The model under review builds one solid part; all positions refer to its coordinate system, in mm. A direction names the side the tool comes from. Give positions to 0.01 mm unless a question says otherwise; leave off trailing zeros. Order: outer loops, then holes, each group sorted by start corner. A loop starts at its lowest first (then second) coordinate and runs counter-clockwise, first axis right, second up. Notation, with made-up numbers: (62.5, 62) - (121.5, 62) arc R18 ccw to (121.5, 66) - close; hole circle Ø7 at (12, -39). An arc over 180 degrees is marked (long way). Put each result on its own line as item: value.
Autodesk Inventor part; units mm, degrees
ref_plane "Work Plane1" through (11.4315, 0, 0) normal (0, 0, -1) x (-1, 0, 0)
ref_plane "YZ Plane" through (0, 0, 0) normal (1, 0, 0) x (0, 1, 0)
ref_plane "XZ Plane" through (0, 0, 0) normal (0, 1, 0) x (-1, 0, 0)
sketch "Skizze1" plane through (0, 0, 0) normal (0, 0, 1) x (1, 0, 0)
  line L0 (-0.8145, 0) -> (4.5691, 0)
  line L1 (1.1089, 2.4) -> (0.7864, 3.6035)
  line L2 (1.1089, 2.4) -> (3.8, 2.4) construction
  line L3 (3.8, 2.4) -> (3.8, 0) construction
  arc A0 (0.7864, 3.6035) -> (0, 3.5) centre (0.4, 3.5) ccw
  line L4 (1.1089, 2.4) -> (1.1089, 0)
  line L5 (0, -0.7897) -> (0, 4.738)
  point P0 (0, 0)
  dimension "d2" = 4.8
  dimension "d4" = 7.8
  dimension "d5" = 0.4
  dimension "d15" = 3.8
  dimension "d16" = 15
revolve "Ring" add sketch "Skizze1" angle 360 about axis through (-10, 0, 0) along (1, 0, 0)
sketch "Skizze2" plane through (0, 0, 0) normal (-1, 0, 0) x (0, 0, 1)
  circle A0 centre (0, 0) radius 4.9
  line L0 (-3, -1.7321) -> (-3, 1.7321)
  line L1 (-3, 1.7321) -> (0, 3.4641)
  line L2 (0, 3.4641) -> (3, 1.7321)
  line L3 (3, 1.7321) -> (3, -1.7321)
  line L4 (3, -1.7321) -> (0, -3.4641)
  line L5 (0, -3.4641) -> (-3, -1.7321)
  dimension "d55" = 6
extrude "Körper" add sketch "Skizze2" against normal blind 3 contours L0 L1 L2 L3 L4 L5
sketch "Skizze3" plane through (0, 0, 0) normal (0, 0, 1) x (1, 0, 0)
  line L0 (0.8237, 3.4641) -> (3, 3.4641)
  line L1 (3, 1.7321) -> (3, 3.4641)
  line L2 (0, -3.5) -> (0, 3.5)
  line L3 (-0.6, 0) -> (3.6, 0)
  line L4 (2.7149, 3.4641) -> (3, 2.4)
  dimension "d10" = 15
  dimension "d11" = 4.8
revolve "Fase1" cut sketch "Skizze3" angle 360 about axis through (-10, 0, 0) along (1, 0, 0)
sketch "Skizze4" plane through (0, 0, 0) normal (-1, 0, 0) x (0, 0, 1)
  circle A0 centre (0, 0) radius 3.5
hole "Gewinde" at (0, 0, 0) direction (1, 0, 0) diameter 2.459 end through all
chamfer "Fase2" distance 0.433 angle 30 1 edges at (0, 0, -1.2295) measured on face at (0, 2.7063, -0.3286)
ref_plane "Work Plane1" through (11.4315, 0, 0) normal (0, 0, -1) x (-1, 0, 0)
chamfer "Fase3" distance 0.433 angle 45 1 edges at (3, 0, -1.2295)
equation "\"d2\" = 0.6 * SW"
equation "\"d16\" = 0.6 * KEWI"
equation "\"d7\" = 0.6 * KOH"
equation "\"d10\" = ANG1"
equation "\"d11\" = 0.6 * SW0"
equation "\"d12\" = -0.5 * GD1 + 0.5 * NND"
equation "\"d46\" = -0.5 * GD1 + 0.5 * NND"
equation "\"d51\" = -0.5 * GD1 + 0.5 * NND"
equation "\"ANG1\" = 15deg"
equation "\"KEWI\" = 25deg"
equation "\"NND\" = 5"
equation "\"LADI\" = 11.8"
equation "\"SW\" = 8"
equation "\"PHH\" = RR"
equation "\"KOH\" = NND"
equation "\"SW0\" = SW"
equation "\"d1\" = LADI"
equation "\"d3\" = PHH"
equation "\"GUL\" = 0.541266 * PTC"
equation "\"RR\" = 1"
equation "\"THREADDIA\" = 5"
equation "\"TOA\" = 30deg"
equation "\"PTC\" = 0.8"
equation "\"GAL\" = 0.541266 * PTC"
equation "\"E0\" = 1.155 * SW"
properties part number "DIN 6923 - M5" material "Stahl, weich"
(1) Take a section at A-A, the plane y = 0. Write out the cut boundary in (x, z), then the cut area to 3 significant figures.
The answers:
outline: (0, -3.5) arc R0.4 ccw to (0.79, -3.6) - (0.95, -3) - (2.84, -3) - (3, -2.4) - (3, -1.66) - (2.57, -1.23) - (0.25, -1.23) - (0, -1.66) - close; (0, 1.66) - (0.25, 1.23) - (2.57, 1.23) - (3, 1.66) - (3, 2.4) - (2.84, 3) - (0.95, 3) - (0.79, 3.6) arc R0.4 ccw to (0, 3.5) - close
area: 11.6 mm^2
(2) For faces 4 (the flat face through (1.8, -2.6, -1.5)), 5 (the flat face through (1.8, 2.6, -1.5)), 6 (the flat face through (1.8, 2.6, 1.5)), list the 3-axis set-ups (+Z, -Z, +X, -X, +Y, -Y) from which the entire face can be reached by the end or side of a thin tool; tool diameter is ignored.
The answers:
face 4: -Z, +X, -Y
face 5: -Z, +X, +Y
face 6: +Z, +X, +Y
(3) Take a section at B-B, the plane x = 2. Write out the cut boundary in (y, z), then the cut area to 3 significant figures.
The answers:
outline: (-3.46, 0) - (-1.73, -3) - (1.73, -3) - (3.46, 0) - (1.73, 3) - (-1.73, 3) - close; hole circle Ø2.46 at (0, 0)
area: 26.4 mm^2
(4) The part is to be moulded in two halves that separate along Z. For faces 1 (the flat face through (3, -2, -1)), 2 (the cylindrical face through (1.425, 0.748, -0.976)), 3 (the flat face through (1.8, -2.6, 1.5)), say which applies: pulls with the +Z half, pulls with the -Z half, needs draft (parallel to the pull), parting line crosses it, or undercut.
The answers:
face 1: needs draft
face 2: undercut
face 3: pulls with the +Z half
(5) Clearance check with flat-ended pins moving along their axes: pin 1 Ø1 at (x, y) = (2, 0) entering from +Z; pin 2 Ø2 at (y, z) = (0, 0) entering from +X (3 decimals); pin 3 Ø1 at (x, z) = (1.5, -2.5) entering from -Y. State where each tip first meets the part, or that it passes through.
The answers:
pin 1: z = 3
pin 2: through
pin 3: y = -2.31
(6) Wall thickness on L1, parallel to Z at x = 2.05, y = 0; L2, parallel to Z at x = 1.3, y = -1.5; L3, parallel to Y at x = 2.6, z = -1: over which ranges is each line inside the solid? List them lowest first.
The answers:
L1: -3 to -1.23, 1.23 to 3
L2: -3 to 3
L3: -2.89 to -0.77, 0.77 to 2.89
